Part model, mm, in its own coordinate system. Round coordinates to 2 decimals unless told otherwise and drop trailing zeros. Write each loop counter-clockwise with the first axis right and the second up, starting at its lowest first coordinate (ties: lowest second). Pieces come first, ordered by that corner, then holes. Notation, with made-up numbers: M 32.5,71 L 68.5,71 A6 cw 68.5,78 Z; hole C 48,23.5 d3. An arc over 180 degrees is marked long. Use one line per item in the form item = value. Start each with the question number.
Item 1: Cut at C-C, the plane x = -9. Give the cut face in (y, z).
Item 2: Cut at B-B, the plane y = 8.75. Give the cut face in (x, z), then the cut area to 3 significant figures.
Item 3: Cut at A-A, the plane x = 0. Give the cut face in (y, z).
Item 4: Flat gauge pins, fed straight in: pin 1 Ø1 at (x, y) = (7, 3) entering from +Z; pin 2 Ø1 at (y, z) = (1.5, 2.5) entering from +X; pin 3 Ø5 at (x, z) = (-2, -3) entering from +Y. Where does each tip first touch, or does it go through?
Item 5: Probe L1, parallel to X at y = 8, z = 0; L2, parallel to Z at x = -1.5, y = 10.25; L3, parallel to X at y = 12.5, z = -4. List the from-to ranges inside material, lowest first.
from build123d import *

# Parameters (mm, degrees)
SKETCH1_R           = 6
EXTRUDE1_DEPTH      = 15
SMUSSO2_SIZE        = 1
SMUSSO3_SIZE        = 0.5
SMUSSO3_EDGE_2_SIZE = 0.5
SMUSSO3_EDGE_3_SIZE = 0.5
SMUSSO3_EDGE_4_SIZE = 0.5
SMUSSO3_EDGE_5_SIZE = 0.5
SMUSSO3_EDGE_6_SIZE = 0.5


with BuildPart() as part:
    # Sketch1 → Extrude1 (new body)
    with BuildSketch(Plane(origin=(0, 0, 0), x_dir=(1, 0, 0), z_dir=(0, 1, 0))):
        Polygon((6.350852961, -11), (12.701705922, 0), (6.350852961, 11), (-6.350852961, 11), (-12.701705922, 0), (-6.350852961, -11), align=None)
        with Locations(Location((0, 0, 0), (0, 0, 270))):
            Circle(SKETCH1_R, mode=Mode.SUBTRACT)
    extrude(amount=EXTRUDE1_DEPTH)

    # Smusso2
    smusso2_edges = [part.edges().sort_by_distance(p)[0] for p in [
        (9.526279442, 15, -5.5),
        (0, 15, -11),
        (0, 0, -6),
        (0, 15, -6),
        (-9.526279442, 15, -5.5),
        (-9.526279442, 15, 5.5),
        (0, 15, 11),
        (-9.526279442, 0, 5.5),
        (-9.526279442, 0, -5.5),
        (0, 0, -11),
        (9.526279442, 0, -5.5),
        (9.526279442, 0, 5.5),
        (0, 0, 11),
        (9.526279442, 15, 5.5),
    ]]
    chamfer(smusso2_edges, length=SMUSSO2_SIZE)

    # Smusso3
    smusso3_edges = [part.edges().sort_by_distance(p)[0] for p in [
        (12.701705922, 7.5, 0),
    ]]
    chamfer(smusso3_edges, length=SMUSSO3_SIZE)

    # Smusso3 edge 2
    smusso3_edge_2_edges = [part.edges().sort_by_distance(p)[0] for p in [
        (6.350852961, 7.5, 11),
    ]]
    chamfer(smusso3_edge_2_edges, length=SMUSSO3_EDGE_2_SIZE)

    # Smusso3 edge 3
    smusso3_edge_3_edges = [part.edges().sort_by_distance(p)[0] for p in [
        (6.350852961, 7.5, -11),
    ]]
    chamfer(smusso3_edge_3_edges, length=SMUSSO3_EDGE_3_SIZE)

    # Smusso3 edge 4
    smusso3_edge_4_edges = [part.edges().sort_by_distance(p)[0] for p in [
        (-6.350852961, 7.5, -11),
    ]]
    chamfer(smusso3_edge_4_edges, length=SMUSSO3_EDGE_4_SIZE)

    # Smusso3 edge 5
    smusso3_edge_5_edges = [part.edges().sort_by_distance(p)[0] for p in [
        (-12.701705922, 7.5, 0),
    ]]
    chamfer(smusso3_edge_5_edges, length=SMUSSO3_EDGE_5_SIZE)

    # Smusso3 edge 6
    smusso3_edge_6_edges = [part.edges().sort_by_distance(p)[0] for p in [
        (-6.350852961, 7.5, 11),
    ]]
    chamfer(smusso3_edge_6_edges, length=SMUSSO3_EDGE_6_SIZE)


solid = part.part
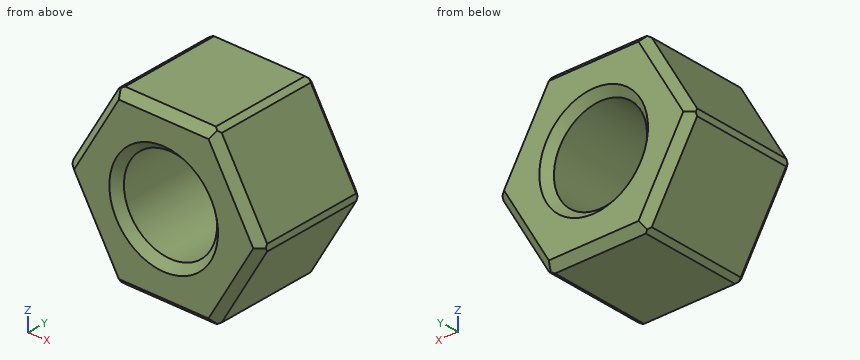
Model answer:
q1.outline = M 0,-4.41 L 1,-6.41 L 14,-6.41 L 15,-4.41 L 15,4.41 L 14,6.41 L 1,6.41 L 0,4.41 Z
q2.outline = M -12.45,-0.43 L -6.6,-10.57 L -5.85,-11 L 5.85,-11 L 6.6,-10.57 L 12.45,-0.43 L 12.45,0.43 L 6.6,10.57 L 5.85,11 L -5.85,11 L -6.6,10.57 L -12.45,0.43 Z; hole C 0,0 d12
q2.area = 305 mm²
q3.outline = M 0,-10 L 1,-11 L 14,-11 L 15,-10 L 15,-7 L 14,-6 L 1,-6 L 0,-7 Z; M 0,7 L 1,6 L 14,6 L 15,7 L 15,10 L 14,11 L 1,11 L 0,10 Z
q4.pin_1 = 10.63
q4.pin_2 = 11.55
q4.pin_3 = 14.11
q5.L1 = -12.45 to -6, 6 to 12.45
q5.L2 = -11 to -5.81, 5.81 to 11
q5.L3 = -10.39 to -4.47, 4.47 to 10.39
